Geometry: see drawing. Coordinates: mm, zero at the bounding-box minimum. A direction names the side the tool comes from. Coordinates: 2 decimals unless noted, no trailing zeros. Order: outer loops, then holes, each group sorted by start corner. A loop starts at its lowest first (then second) coordinate and runs counter-clockwise, first axis right, second up. Notation, with made-up numbers: (54, -26) -> (83, -26) arc R21 ccw to (83, 4) -> close; hole circle Ø1 at (60.25, 88.25). An arc over 180 degrees is marked (long way). Write each question's results on one line, items separated by ' | '.
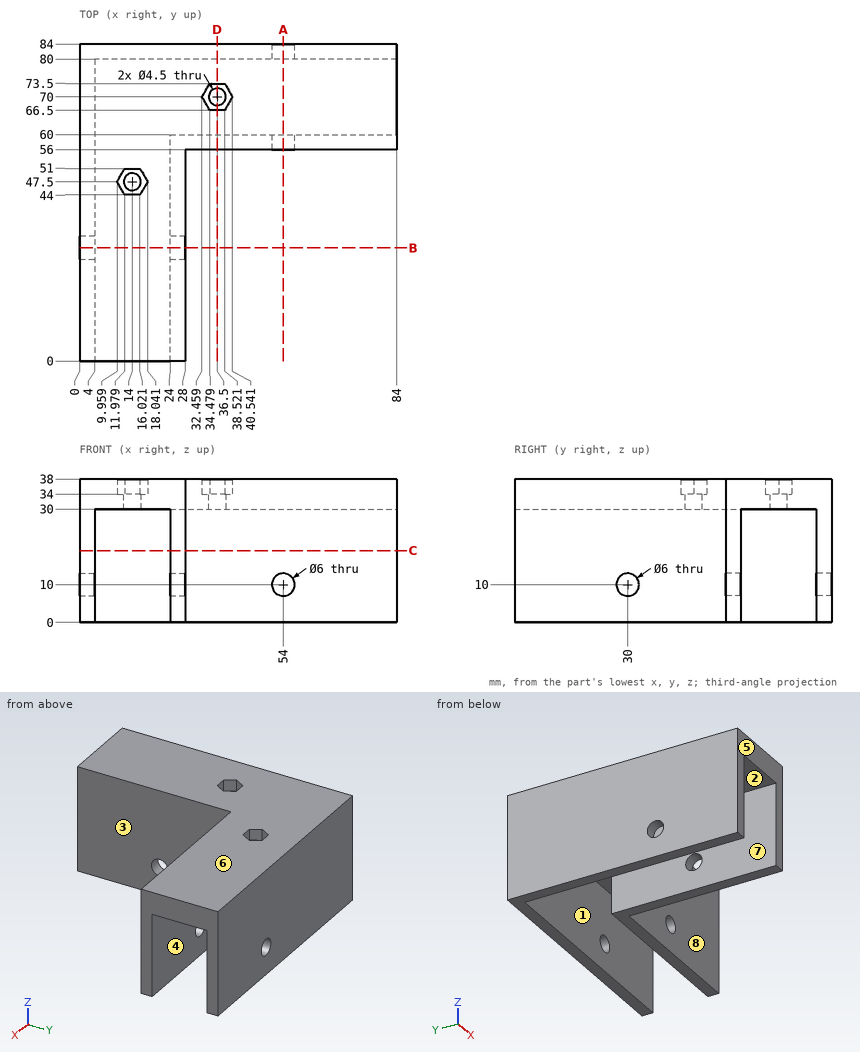
(1) Pin query (flat end, axial travel): P1, Ø6, axis at x = 36.5, y = 70, coming from the +Z side; P2, Ø1.2, axis at x = 35.5, z = 36.5, coming from the -Y side; P3, Ø9.5, axis at y = 30, z = 10, coming from the +X side; P4, Ø5.5, axis at x = 54, z = 10, coming from the -Y side. Return the tip coordinate at first contact, or that it passes through.
Return value:
P1: z = 34 | P2: y = 56 | P3: x = 28 | P4: through
(2) Cut plane A-A, the plane x = 54. Return loops of the section in (y, z).
Return value:
outline: (56, 0) -> (60, 0) -> (60, 7) -> (56, 7) -> close; (56, 13) -> (60, 13) -> (60, 30) -> (80, 30) -> (80, 13) -> (84, 13) -> (84, 38) -> (56, 38) -> close; (80, 0) -> (84, 0) -> (84, 7) -> (80, 7) -> close
(3) Cut plane C-C, the plane z = 19. Return loops of the section in (x, y), plus the area to 3 significant figures.
Return value:
outline: (0, 0) -> (4, 0) -> (4, 80) -> (84, 80) -> (84, 84) -> (0, 84) -> close; (24, 0) -> (28, 0) -> (28, 56) -> (84, 56) -> (84, 60) -> (24, 60) -> close | area: 1,120 mm2
(4) Reachability of the marked faces 4, 5, 6, 7 and 8 from +Z, -Z, +X, -X, +Y, -Y: full face, straight path, thin tool, end or side. Return the list, or none.
Return value:
face 4: -Z, +X | face 5: +Z, -Z, +X, -X, -Y | face 6: +Z, +X, -X, +Y, -Y | face 7: -Z, -Y | face 8: +Z, -Z, +X, -Y
(5) Cut plane D-D, the plane x = 36.5. Return loops of the section in (y, z), plus the area to 3 significant figures.
Return value:
outline: (56, 0) -> (60, 0) -> (60, 30) -> (67.75, 30) -> (67.75, 34) -> (66.5, 34) -> (66.5, 38) -> (56, 38) -> close; (72.25, 30) -> (80, 30) -> (80, 0) -> (84, 0) -> (84, 38) -> (73.5, 38) -> (73.5, 34) -> (72.25, 34) -> close | area: 418 mm2
(6) Cut plane B-B, the plane y = 30. Return loops of the section in (x, z), plus the area to 3 significant figures.
Return value:
outline: (0, 0) -> (4, 0) -> (4, 7) -> (0, 7) -> close; (0, 13) -> (4, 13) -> (4, 30) -> (24, 30) -> (24, 13) -> (28, 13) -> (28, 38) -> (0, 38) -> close; (24, 0) -> (28, 0) -> (28, 7) -> (24, 7) -> close | area: 416 mm2
(7) Mould query, pull axis X, two halves, no side actions, for the marked faces 1, 2 and 3. Classes: +X half, -X half, draft (parallel to the pull), parting line (faces both ways), or undercut.
Return value:
face 1: draft | face 2: undercut | face 3: +X half
(8) Line query: line 1 along Y through (x, z) = (46, 4); line 2 along Z through (x, y) = (54, 57.6); line 3 along X through (y, z) = (31, 20.5). Output: solid intervals per line, ascending. Write a range as from..to.
Return value:
line 1: 56..60, 80..84 | line 2: 0..7, 13..38 | line 3: 0..4, 24..28
